from build123d import *

# Parameters (mm, degrees)
F0_R     = 5
F0_R_2   = 2
F1_DEPTH = 8
F3_DEPTH = 3
F5_DEPTH = 210
F7_DEPTH = 190


with BuildPart() as f1:
    # F0 (on Top) → F1 (new body)
    with BuildSketch(Plane.XY):
        with BuildLine():
            ThreePointArc((3.9848484304, 22.652173913), (0, 27), (-3.9848484304, 22.652173913))
            ThreePointArc((-3.9848484304, 22.652173913), (-23, 0), (-3.9848484304, -22.652173913))
            ThreePointArc((-3.9848484304, -22.652173913), (0, -27), (3.9848484304, -22.652173913))
            ThreePointArc((3.9848484304, -22.652173913), (23, 0), (3.9848484304, 22.652173913))
        make_face()
        Circle(F0_R, mode=Mode.SUBTRACT)
        with Locations((8, 0)):
            Circle(F0_R_2, mode=Mode.SUBTRACT)
    extrude(amount=F1_DEPTH)

    # F2 (on face) → F3 (cut)
    with BuildSketch(Plane.XY.offset(8)):
        with BuildLine():
            ThreePointArc((-3.9848484304, 22.652173913), (0, 23), (3.9848484304, 22.652173913))
            ThreePointArc((3.9848484304, 22.652173913), (0, 27), (-3.9848484304, 22.652173913))
        make_face()
        with BuildLine():
            ThreePointArc((-3.9848484304, -22.652173913), (0, -27), (3.9848484304, -22.652173913))
            ThreePointArc((3.9848484304, -22.652173913), (0, -23), (-3.9848484304, -22.652173913))
        make_face()
    extrude(amount=-F3_DEPTH, mode=Mode.SUBTRACT)

    # F4 (on face) → F5 (join)
    with BuildSketch(Plane(origin=(0, 0, 0), x_dir=(1, 0, 0), z_dir=(0, 0, -1))):
        with BuildLine():
            Line((-2, -4.582575695), (-2, -24))
            Line((-2, -24), (2, -24))
            Line((2, -24), (2, -4.582575695))
            ThreePointArc((2, -4.582575695), (0, -5), (-2, -4.582575695))
        make_face()
        with BuildLine():
            Line((-2, 24), (-2, 4.582575695))
            ThreePointArc((-2, 4.582575695), (0, 5), (2, 4.582575695))
            Line((2, 4.582575695), (2, 24))
            Line((2, 24), (-2, 24))
        make_face()
    extrude(amount=F5_DEPTH)

    # F6 (on face) → F7 (join)
    with BuildSketch(Plane(origin=(0, 0, -210), x_dir=(1, 0, 0), z_dir=(0, 0, -1))):
        with BuildLine():
            ThreePointArc((2, 4.582575695), (0, 5), (-2, 4.582575695))
            Line((-2, 4.582575695), (-2, -4.582575695))
            ThreePointArc((-2, -4.582575695), (0, -5), (2, -4.582575695))
            Line((2, -4.582575695), (2, 4.582575695))
        make_face()
    extrude(amount=-F7_DEPTH)


solid = f1.part
Could you check a few things on this model? Use its own coordinates, in mm. A direction names the side the tool comes from. Give positions to 0.01 mm unless a question says otherwise; leave off trailing zeros. Order: outer loops, then holes, each group sorted by start corner. A loop starts at its lowest first (then second) coordinate and runs counter-clockwise, first axis right, second up.
Item 1: If we section it at C-C, the plane z = -88: Write out the boundary of the cut face in (x, y).
Item 2: If we section it at D-D, the plane x = -11: Write out the boundary of the cut face in (y, z).
Item 3: I need wall thicknesses on line 1 (Y direction, x = 0, z = 3.25); line 2 (X direction, y = -11.5, z = -65); line 3 (Z direction, x = 1, y = 4.5). Which ranges of each line are inside material? Lowest first, please.
Item 4: If we section it at B-B, the plane y = 19: Write out the boundary of the cut face in (x, z), plus the area to 3 significant figures.
Item 5: If we mould it in two halves opening along Y, with no side actions, what happens to faces 1 (the face through (6, 0, 4)), 2 (the face through (0, 24, -104)), 3 (the face through (0, 0, -20)), 4 (the face through (0, 0, -210))? For each: pulls with the +Y half, pulls with the -Y half, needs draft (parallel to the pull), parting line crosses it, or undercut.
Item 6: I'm going to push flat-ended pins straight in: pin 1 (14.5 mm diameter, centred on y = 1, z = -55, fed in from -X); pin 2 (1 mm diameter, centred on y = -7.5, z = -60, fed in from +X); pin 3 (3 mm diameter, centred on x = 0, y = -2, fed in from +Z). Where does each tip first touch, or does it pass through?
Item 7: For faces 5 (the face through (2, 0, -106)), 6 (the face through (0, -24, -104)), 7 (the face through (-5.4, 0.3, 8)), 8 (the face through (-2, 0, -106)), which set-ups out of +Z, -Z, +X, -X, +Y, -Y let a thin tool reach every point of the face, with its end or its side?
Item 8: If we section it at A-A, the plane x = 8: Write out the boundary of the cut face in (y, z).
Values:
1. outline: (-2, -24) - (2, -24) - (2, 24) - (-2, 24) - close
2. outline: (-20.2, 0) - (20.2, 0) - (20.2, 8) - (-20.2, 8) - close
3. line 1: y = -27 to -5, 5 to 27
3. line 2: x = -2 to 2
3. line 3: z = -210 to -20
4. outline: (-12.96, 0) - (-2, 0) - (-2, -210) - (2, -210) - (2, 0) - (12.96, 0) - (12.96, 8) - (-12.96, 8) - close
4. area: 1,050 mm2
5. face 1: undercut
5. face 2: pulls with the +Y half
5. face 3: undercut
5. face 4: needs draft
6. pin 1: stops at x = -2
6. pin 2: stops at x = 2
6. pin 3: stops at z = -20
7. face 5: -Z, +X, +Y, -Y
7. face 6: -Z, +X, -X, -Y
7. face 7: +Z, +X, -X, +Y, -Y
7. face 8: -Z, -X, +Y, -Y
8. outline: (-21.56, 0) - (-2, 0) - (-2, 8) - (-21.56, 8) - close; (2, 0) - (21.56, 0) - (21.56, 8) - (2, 8) - close
